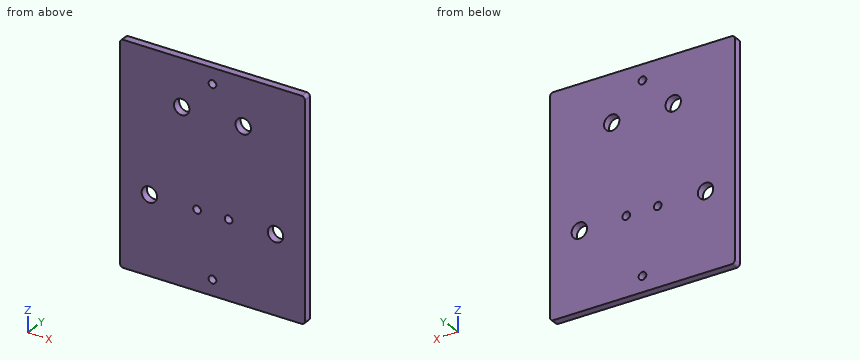
```python
from build123d import *

# Parameters (mm, degrees)
SKETCH1_W           = 152.4
SKETCH1_H           = 177.8
SKETCH1_R           = 6.35
SKETCH1_R_2         = 3.175
BOSS_EXTRUDE1_DEPTH = 6.35
FILLET1_R           = 2.54


with BuildPart() as part:
    # Sketch1 → Boss-Extrude1 (new body)
    with BuildSketch(Plane(origin=(0, 0, 0), x_dir=(1, 0, 0), z_dir=(0, 1, 0))):
        with Locations((76.2, 88.9)):
            Rectangle(SKETCH1_W, SKETCH1_H)
        with Locations((24.13, 114.3)):
            Circle(SKETCH1_R, mode=Mode.SUBTRACT)
        with Locations((128.27, 114.3)):
            Circle(SKETCH1_R, mode=Mode.SUBTRACT)
        with Locations((50.8, 38.1)):
            Circle(SKETCH1_R, mode=Mode.SUBTRACT)
        with Locations((101.6, 38.1)):
            Circle(SKETCH1_R, mode=Mode.SUBTRACT)
        with Locations((76.2, 165.1)):
            Circle(SKETCH1_R_2, mode=Mode.SUBTRACT)
        with Locations((76.2, 12.7)):
            Circle(SKETCH1_R_2, mode=Mode.SUBTRACT)
        with Locations((63.5, 114.3)):
            Circle(SKETCH1_R_2, mode=Mode.SUBTRACT)
        with Locations((89.535, 114.3)):
            Circle(SKETCH1_R_2, mode=Mode.SUBTRACT)
    extrude(amount=BOSS_EXTRUDE1_DEPTH)

    # Fillet1
    fillet1_edges = [part.edges().sort_by_distance(p)[0] for p in [
        (0, 3.175, -177.8),
        (152.4, 3.175, -177.8),
        (152.4, 3.175, 0),
        (0, 3.175, 0),
    ]]
    fillet(fillet1_edges, radius=FILLET1_R)


solid = part.part
```
Can you work these out from the model? Positions are in its coordinate system, mm. Round coordinates to 2 decimals unless told otherwise and drop trailing zeros. Order: outer loops, then holes, each group sorted by start corner. A loop starts at its lowest first (then second) coordinate and runs counter-clockwise, first axis right, second up.
(1) If I drill on L1, parallel to X at y = 4.75, z = -114.3 (3 decimals); L2, parallel to X at y = 5, z = -38.1; L3, parallel to Z at x = 24.13, y = 4.75, over which ranges is the centre line in solid material (lowest first)?
Results are:
L1: x = 0 to 17.78, 30.48 to 60.325, 66.675 to 86.36, 92.71 to 121.92, 134.62 to 152.4
L2: x = 0 to 44.45, 57.15 to 95.25, 107.95 to 152.4
L3: z = -177.8 to -120.65, -107.95 to 0
(2) If we section it at A-A (z = -114.3): Please give me the cut outline in (x, y) (3 decimals), plus the area to 3 significant figures.
Results are:
outline: (0, 0) - (17.78, 0) - (17.78, 6.35) - (0, 6.35) - close; (30.48, 0) - (60.325, 0) - (60.325, 6.35) - (30.48, 6.35) - close; (66.675, 0) - (86.36, 0) - (86.36, 6.35) - (66.675, 6.35) - close; (92.71, 0) - (121.92, 0) - (121.92, 6.35) - (92.71, 6.35) - close; (134.62, 0) - (152.4, 0) - (152.4, 6.35) - (134.62, 6.35) - close
area: 726 mm2
(3) If we section it at B-B (x = 128.27): Please give me the cut outline in (y, z), plus the area to 3 significant figures.
Results are:
outline: (0, -177.8) - (6.35, -177.8) - (6.35, -120.65) - (0, -120.65) - close; (0, -107.95) - (6.35, -107.95) - (6.35, 0) - (0, 0) - close
area: 1,050 mm2
(4) If we section it at D-D (y = 4.25): Count the separate pieces of the cut face and the enclosed holes in it, plus the area to 3 significant figures.
Results are:
separate pieces: 1
enclosed holes: 8
area: 26,500 mm2
(5) I'm going to push a flat-ended pin straight in: pin 1 (11.5 mm diameter, centred on x = 128.27, z = -114.3, fed in from +Y). Where does the tip first touch, or does it pass through?
Results are:
pin 1: passes through
(6) If we section it at C-C (z = -165.1): Please give me the cut outline in (x, y) (3 decimals).
Results are:
outline: (0, 0) - (73.025, 0) - (73.025, 6.35) - (0, 6.35) - close; (79.375, 0) - (152.4, 0) - (152.4, 6.35) - (79.375, 6.35) - close
